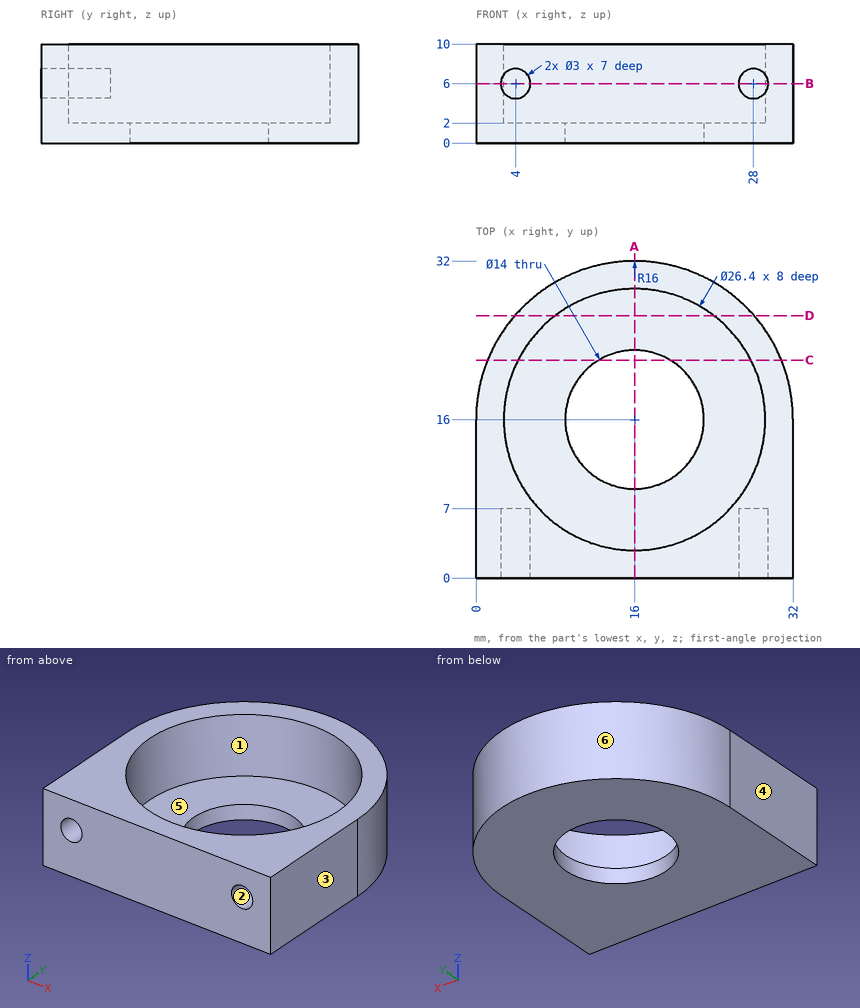
The figure shows three views and two pictorial views of one solid part (mm, origin at its lowest corner). Answer the questions. A direction names the side the tool comes from. Coordinates: 2 decimals unless noted, no trailing zeros. Loops run counter-clockwise (first coordinate to the right, second up) from the corner with the lowest first, then second, coordinate; pieces in that order, holes last.
1) Flat-ended cylindrical pins translate along their axes: pin 1 Ø0.9 at (x, z) = (27.5, 6) entering from -Y; pin 2 Ø6 at (y, z) = (26.5, 4.5) entering from -X; pin 3 Ø1 at (x, y) = (13, 5.5) entering from +Z; pin 4 Ø12.5 at (x, y) = (16, 16) entering from +Z. Find the tip coordinate at first contact, or state that the pin passes through.
2) Find section C-C on y = 22. Write down the section's boundary in (x, z), then the cut area to 3 significant figures.
3) Find section B-B on z = 6. Write down the section's boundary in (x, y).
4) Find section D-D on y = 26.5. Write down the section's boundary in (x, z), then the cut area to 3 significant figures.
5) Find the intervals of material crossed by L1, parallel to Z at x = 4, y = 5.25; L2, parallel to Y at x = 16, z = 0.6; L3, parallel to Y at x = 16, z = 7.5, in increasing order.
6) Determine the mould class of the marked faces 4, 5 and 6 for opening direction Y: pulls with the +Y half, pulls with the -Y half, needs draft (parallel to the pull), parting line crosses it, or undercut.
7) Find section A-A on x = 16. Write down the section's boundary in (y, z).
8) A tool of negligible diameter and unlimited length cuts with its end or side. For the marked faces 1, 2 and 3, from which of +Z, -Z, +X, -X, +Y, -Y can it reach the whole face along a straight path? Write none if from no direction.
Values:
1. pin 1: stops at y = 7
1. pin 2: stops at x = 1.87
1. pin 3: stops at z = 2
1. pin 4: passes through
2. outline: (1.17, 0) - (12.39, 0) - (12.39, 2) - (4.24, 2) - (4.24, 10) - (1.17, 10) - close; (19.61, 0) - (30.83, 0) - (30.83, 10) - (27.76, 10) - (27.76, 2) - (19.61, 2) - close
2. area: 94.1 mm2
3. outline: (0, 0) - (2.5, 0) - (2.5, 7) - (5.5, 7) - (5.5, 0) - (26.5, 0) - (26.5, 7) - (29.5, 7) - (29.5, 0) - (32, 0) - (32, 16) arc R16 ccw to (0, 16) - close; hole circle Ø26.4 at (16, 16)
4. outline: (3.93, 0) - (28.07, 0) - (28.07, 10) - (24, 10) - (24, 2) - (8, 2) - (8, 10) - (3.93, 10) - close
4. area: 113 mm2
5. L1: z = 0 to 4.5, 7.5 to 10
5. L2: y = 0 to 9, 23 to 32
5. L3: y = 0 to 2.8, 29.2 to 32
6. face 4: needs draft
6. face 5: undercut
6. face 6: pulls with the +Y half
7. outline: (0, 0) - (9, 0) - (9, 2) - (2.8, 2) - (2.8, 10) - (0, 10) - close; (23, 0) - (32, 0) - (32, 10) - (29.2, 10) - (29.2, 2) - (23, 2) - close
8. face 1: +Z
8. face 2: -Y
8. face 3: +Z, -Z, +X, +Y, -Y
